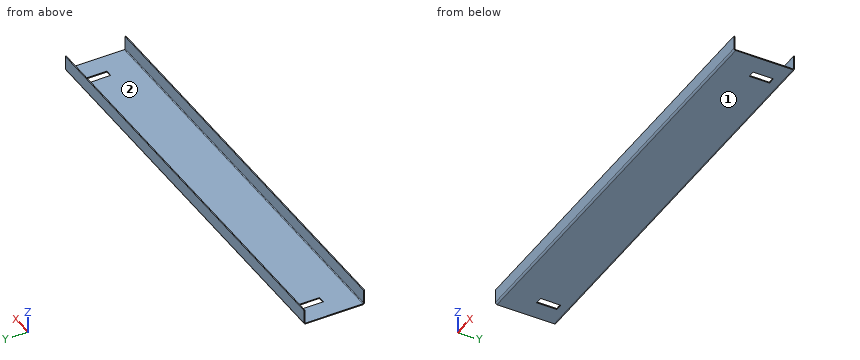
from build123d import *

# Parameters (mm, degrees)
SKETCH1_W                    = 420
SKETCH1_H                    = 60
BASE_FLANGE1_DEPTH           = 1
EDGE_FLANGE1_STRIP_W         = 5.4732
EDGE_FLANGE1_STRIP_H         = 1
EDGE_FLANGE1_STRIP_CUT_DEPTH = 420
EDGE_FLANGE1_DEPTH           = 420
EDGE_FLANGE2_STRIP_W         = 5.4732
EDGE_FLANGE2_STRIP_H         = 1
EDGE_FLANGE2_STRIP_CUT_DEPTH = 420
EDGE_FLANGE2_DEPTH           = 420
SKETCH12_W                   = 7
SKETCH12_H                   = 20
CUT_EXTRUDE1_DEPTH           = 217.028384653


# Sheet-metal steps are written as plain solids
with BuildPart() as part:
    # Sketch1 → Base-Flange1 (new body)
    with BuildSketch(Plane.XY):
        with Locations((0, 18.705882353)):
            Rectangle(SKETCH1_W, SKETCH1_H)
    extrude(amount=-BASE_FLANGE1_DEPTH)

    # Edge-Flange1 strip (across the edge) → Edge-Flange1 strip cut (cut)
    with BuildSketch(Plane(origin=(210, 48.705882353, 0), x_dir=(0, -1, 0), z_dir=(-1, 0, 0))):
        with Locations((-1, -0.5)):
            Rectangle(EDGE_FLANGE1_STRIP_W, EDGE_FLANGE1_STRIP_H)
    extrude(amount=EDGE_FLANGE1_STRIP_CUT_DEPTH, mode=Mode.SUBTRACT)

    # Edge-Flange1 section (across the edge) → Edge-Flange1 (add)
    with BuildSketch(Plane(origin=(210, 48.705882353, 0), x_dir=(0, -1, 0), z_dir=(-1, 0, 0))):
        with BuildLine():
            Line((0, 0.7366), (0, 14))
            Line((0, 14), (1, 14))
            Line((1, 14), (1, 0.7366))
            ThreePointArc((1, 0.7366), (1.215745145, 0.215745145), (1.7366, 0))
            Line((1.7366, 0), (1.7366, -1))
            ThreePointArc((1.7366, -1), (0.508638364, -0.491361636), (0, 0.7366))
        make_face()
    extrude(amount=EDGE_FLANGE1_DEPTH)

    # Edge-Flange2 strip (across the edge) → Edge-Flange2 strip cut (cut)
    with BuildSketch(Plane(origin=(-210, -11.294117647, 0), x_dir=(0, 1, 0), z_dir=(1, 0, 0))):
        with Locations((-1, -0.5)):
            Rectangle(EDGE_FLANGE2_STRIP_W, EDGE_FLANGE2_STRIP_H)
    extrude(amount=EDGE_FLANGE2_STRIP_CUT_DEPTH, mode=Mode.SUBTRACT)

    # Edge-Flange2 section (across the edge) → Edge-Flange2 (add)
    with BuildSketch(Plane(origin=(-210, -11.294117647, 0), x_dir=(0, 1, 0), z_dir=(1, 0, 0))):
        with BuildLine():
            Line((0, 0.7366), (0, 14))
            Line((0, 14), (1, 14))
            Line((1, 14), (1, 0.7366))
            ThreePointArc((1, 0.7366), (1.215745145, 0.215745145), (1.7366, 0))
            Line((1.7366, 0), (1.7366, -1))
            ThreePointArc((1.7366, -1), (0.508638364, -0.491361636), (0, 0.7366))
        make_face()
    extrude(amount=EDGE_FLANGE2_DEPTH)

    # Sketch12 → Cut-Extrude1 (cut, through all)
    with BuildSketch(Plane.XY):
        with Locations((186.818027369, 28.75)):
            Rectangle(SKETCH12_W, SKETCH12_H)
        with Locations((-187.355, 28.75)):
            Rectangle(SKETCH12_W, SKETCH12_H)
    extrude(amount=-CUT_EXTRUDE1_DEPTH, mode=Mode.SUBTRACT)


solid = part.part
Read the model definition and answer for the solid it produces. Units are mm, in the model's axes. Face numbers are marked on the shaded views. A direction names the side the tool comes from. Round coordinates to 2 decimals unless told otherwise and drop trailing zeros. Write each loop counter-clockwise with the first axis right and the second up, starting at its lowest first coordinate (ties: lowest second). Pieces come first, ordered by that corner, then holes.
Q1. Flat-ended cylindrical pins translate along their axes: P1, Ø0.8, axis at x = 185, z = -0.5, coming from the +Y side; P2, Ø3, axis at x = 88.5, y = 10.5, coming from the +Z side; P3, Ø1.1, axis at x = -187, z = -0.5, coming from the -Y side. Find the tip coordinate at first contact, or state that the pin passes through.
Values:
P1: stops at y = 48.49
P2: stops at z = 0
P3: stops at y = -11.15
Q2. A tool of negligible diameter and unlimited length cuts with its end or side. For the marked faces 1 and 2, from which of +Z, -Z, +X, -X, +Y, -Y can it reach the whole face along a straight path? Write none if from no direction.
Values:
face 1: -Z, +X, -X, +Y, -Y
face 2: +Z, +X, -X
Q3. Find section B-B on x = 5. Determine the outline of the cut face in (y, z).
Values:
outline: (-11.29, 0.74) arc R1.74 ccw to (-9.56, -1) - (46.97, -1) arc R1.74 ccw to (48.71, 0.74) - (48.71, 14) - (47.71, 14) - (47.71, 0.74) arc R0.74 cw to (46.97, 0) - (-9.56, 0) arc R0.74 cw to (-10.29, 0.74) - (-10.29, 14) - (-11.29, 14) - close
Q4. Find section A-A on z = 6.75. Determine the outline of the cut face in (x, y), and give its area (3 significant figures).
Values:
outline: (-210, -11.29) - (210, -11.29) - (210, -10.29) - (-210, -10.29) - close; (-210, 47.71) - (210, 47.71) - (210, 48.71) - (-210, 48.71) - close
area: 840 mm2
Q5. Straight lines are drawn through the part: line 1 (Y direction, x = 34.5, z = 10.75); line 2 (Z direction, x = 127, y = 7); line 3 (Y direction, x = 124.5, z = 0.25). For each, find the intervals that lie inside material, in ascending order.
Values:
line 1: y = -11.29 to -10.29, 47.71 to 48.71
line 2: z = -1 to 0
line 3: y = -11.22 to -10.11, 47.52 to 48.64
